Design review of the part built by this model. Coordinates are the model's own, in mm. A direction names the side the tool comes from. Coordinates: 2 decimals unless noted, no trailing zeros. Write each loop counter-clockwise with the first axis right and the second up, starting at its lowest first coordinate (ties: lowest second). Pieces come first, ordered by that corner, then holes. Notation, with made-up numbers: M 56,-5 L 80,-5 A30 cw 80,28 Z; hole C 26.5,59 d9. An arc over 180 degrees is marked long. Write item = value, one per line.
```python
from build123d import *

# Parameters (mm, degrees)
F0_W     = 26.6
F0_H     = 11.5
F1_DEPTH = 11.5
F2_W     = 5.8
F2_H     = 7
F2_W_2   = 10
F2_H_2   = 8
F3_DEPTH = 5.751


with BuildPart() as f1:
    # F0 (on Top) → F1 (new body)
    with BuildSketch(Plane.XY):
        Rectangle(F0_W, F0_H)
    extrude(amount=F1_DEPTH)

    # F2 (on Front) → F3 (cut, through all)
    with BuildSketch(Plane.XZ):
        with Locations((-10.4, 8)):
            Rectangle(F2_W, F2_H)
        with Locations((10.4, 8)):
            Rectangle(F2_W, F2_H)
        with Locations((0, 4)):
            Rectangle(F2_W_2, F2_H_2)
    extrude(amount=F3_DEPTH, mode=Mode.SUBTRACT)


solid = f1.part
```
Q1. Consider section A-A, the plane x = 0. State the section outline as (y, z) points.
Check result:
outline = M -5.75,8 L 0,8 L 0,0 L 5.75,0 L 5.75,11.5 L -5.75,11.5 Z
Q2. Consider section C-C, the plane z = 6.25. State the section outline as (x, y) points.
Check result:
outline = M -13.3,0 L -7.5,0 L -7.5,-5.75 L -5,-5.75 L -5,0 L 5,0 L 5,-5.75 L 7.5,-5.75 L 7.5,0 L 13.3,0 L 13.3,5.75 L -13.3,5.75 Z
Q3. Machinability: for faces 1 (the flat face through (-10, -3, 4.5)), 2 (the flat face through (10, 0, 8)), 3 (the flat face through (0, 1, 0)), 4 (the flat face through (5, -3, 4)), which of the approach directions +Z, -Z, +X, -X, +Y, -Y give a long, thin tool a straight path to every point of the face, cutting with its end or side? Answer none if there is none.
Check result:
face_1 = +Z, -X, -Y
face_2 = +Z, +X, -Y
face_3 = -Z, +X, -X, +Y, -Y
face_4 = -Z, -Y
Q4. Consider section D-D, the plane z = 1. State the section outline as (x, y) points.
Check result:
outline = M -13.3,-5.75 L -5,-5.75 L -5,0 L 5,0 L 5,-5.75 L 13.3,-5.75 L 13.3,5.75 L -13.3,5.75 Z
Q5. Wall thickness on line 1 (X direction, y = -2, z = 6); line 2 (Z direction, x = -2.5, y = -2.5); line 3 (Y direction, x = -10.25, z = 10.25): over which ranges is each line inside the solid? List them lowest first.
Check result:
line_1 = -7.5 to -5, 5 to 7.5
line_2 = 8 to 11.5
line_3 = 0 to 5.75
Q6. For P1, Ø4.5, axis at y = -3, z = 9.5, coming from the +X side; P2, Ø3, axis at x = -1.5, y = -3, coming from the -Z side; P3, Ø5, axis at x = 10.5, z = 7.5, coming from the -Y side; P4, Ø1.5, axis at x = 5.5, y = 4, coming from the -Z side, all flat-tipped, find the tip position at first contact; note any pin that passes through.
Check result:
P1 = 7.5
P2 = 8
P3 = 0
P4 = 0
Q7. Consider section B-B, the plane y = -1. State the section outline as (x, z) points.
Check result:
outline = M -13.3,0 L -5,0 L -5,8 L 5,8 L 5,0 L 13.3,0 L 13.3,4.5 L 7.5,4.5 L 7.5,11.5 L -7.5,11.5 L -7.5,4.5 L -13.3,4.5 Z
Q8. The part is to be moulded in two halves that separate along X. For faces 5 (the flat face through (7.5, -3, 8)), 6 (the flat face through (-0.2, -5.75, 8.2)), 7 (the flat face through (0, 0, 4)), say which applies: +X half, -X half, draft (parallel to the pull), parting line (faces both ways), or undercut.
Check result:
face_5 = +X half
face_6 = draft
face_7 = undercut
